Geometry: final body of the model. Coordinates: model frame, mm. Face numbers are marked on the shaded views. A direction names the side the tool comes from. Coordinates: 2 decimals unless noted, no trailing zeros. Order: outer loops, then holes, each group sorted by start corner. A loop starts at its lowest first (then second) coordinate and runs counter-clockwise, first axis right, second up. Notation, with made-up numbers: M 78,22.5 L 131,22.5 A19 cw 131,37.5 Z; hole C 19.5,51 d6. An arc over 180 degrees is marked long. Use CSV: the item, a comma, the result in double quotes. Start each with the question number.
Q1. Mould query, pull axis Y, two halves, no side actions, for the marked faces 4, 5, 6 and 7. Classes: +Y half, -Y half, draft (parallel to the pull), parting line (faces both ways), or undercut.
Q2. Section query B-B, the plane y = -1.5. Output: boundary loops of the cut face in (x, z), and give its area (3 significant figures).
Q3. Section query A-A, the plane x = -17. Output: boundary loops of the cut face in (y, z).
Q4. Access query for the marked faces 1, 2 and 3. Directions: +Z, -Z, +X, -X, +Y, -Y. A direction counts if a zero-diameter tool reaches every point of the face in a straight line with its end or side. Return the directions, or none.
Q5. Ray query, probe 1 along Z at (x, y) = (23, -24); probe 2 along X at (y, z) = (0, 9.25); probe 3 along X at (y, z) = (-14.5, 8.5). Return the intervals inside material, ascending.
Q6. First-contact query: P1, Ø2.5, axis at x = 23, z = 7, coming from the +Y side; P2, Ø1, axis at x = 7.5, z = 1.5, coming from the -Y side; P3, Ø2, axis at x = 12.03, y = 7.16, coming from the -Z side; P4, Ø3, axis at y = 8, z = 8.5, coming from the -X side. Flat tips, straight axial feed; report the tip coordinate or a pass-through.
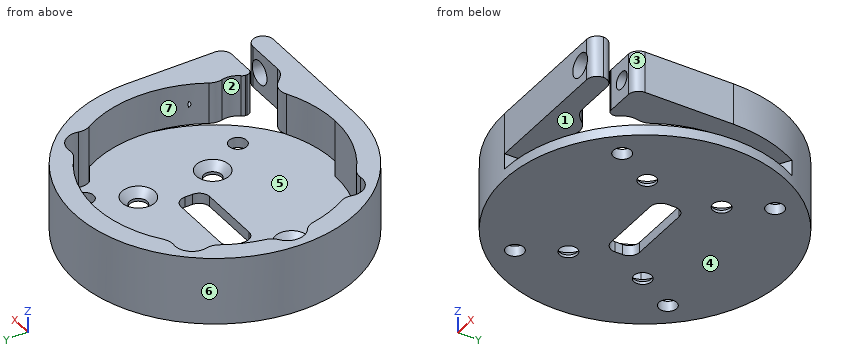
from build123d import *

# Parameters (mm, degrees)
SKETCH_1_R                   = 27
SKETCH_1_R_2                 = 23.1
EXTRUDE_1_DEPTH              = 11
EXTRUDE_START                = 2
SKETCH_2_R                   = 27
EXTRUDE_2_DEPTH              = 2
EXTRUDE_START_2              = -8
EXTRUDE_3_DEPTH              = 8
CUT_EXTRUDE_START            = -8
CUT_EXTRUDE_1_DEPTH          = 8
HOLE_WIZARD_M41_D            = 4.5
HOLE_WIZARD_M41_DEPTH        = 3.9
M4X0_71_D                    = 3.3
M4X0_71_DEPTH                = 10.5
M4X0_71_TIP                  = 0.991420021
CUT_EXTRUDE_START_2          = -3
CUT_EXTRUDE_2_DEPTH          = 3
FILLET_1_R                   = 2
SKETCH_11_W                  = 16
SKETCH_11_H                  = 5.5
CUT_EXTRUDE_3_DEPTH          = 40.736633068
SKETCH_15_R                  = 3.3
SKETCH_15_R_2                = 3.5
CUT_EXTRUDE_5_DEPTH          = 40.736633068
FILLET_3_R                   = 3
SKETCH_16_W                  = 6.088373552
SKETCH_16_H                  = 3.13806494
CUT_EXTRUDE_6_DEPTH          = 11
HOLE_WIZARD_M31_D            = 3.4
HOLE_WIZARD_M31_DEPTH        = 18
HOLE_WIZARD_M31_TIP          = 1.021463052
HOLE_WIZARD_M31_2_AT_2_COUNT = 2
HOLE_WIZARD_M31_2_AT_2_PITCH = 14.310111001
HOLE_WIZARD_M31_2_AT_3_COUNT = 2
HOLE_WIZARD_M31_2_AT_3_PITCH = 28
HOLE_WIZARD_M31_2_AT_4_COUNT = 2
HOLE_WIZARD_M31_2_AT_4_PITCH = 24.067004865
FILLET_7_R                   = 2
EXTRUDE_4_DEPTH              = 8
FILLET_8_R                   = 3
FILLET_9_R                   = 1


with BuildPart() as part:
    # Эскиз1 → Бобышка-Вытянуть1 (new body)
    with BuildSketch(Plane.XY):
        Circle(SKETCH_1_R)
        Circle(SKETCH_1_R_2, mode=Mode.SUBTRACT)
    extrude(amount=EXTRUDE_1_DEPTH)

    # Эскиз2 → Бобышка-Вытянуть2 (add)
    with BuildSketch(Plane(origin=(0, 0, 0), x_dir=(-1, 0, 0), z_dir=(0, 0, -1)).offset(EXTRUDE_START)):
        Circle(SKETCH_2_R)
    extrude(amount=-EXTRUDE_2_DEPTH)

    # Эскиз3 → Бобышка-Вытянуть3 (add)
    with BuildSketch(Plane.XY.offset(11).offset(EXTRUDE_START_2)):
        with BuildLine():
            Line((0, -27), (27, -27))
            Line((27, -27), (27, 0))
            ThreePointArc((27, 0), (19.091883092, -19.091883092), (0, -27))
        make_face()
    extrude(amount=EXTRUDE_3_DEPTH)

    # Эскиз4 → Вырез-Вытянуть1 (cut)
    with BuildSketch(Plane.XY.offset(11).offset(CUT_EXTRUDE_START)):
        with BuildLine():
            Line((0, -23.1), (27, -23.1))
            Line((27, -23.1), (27, -19))
            Line((27, -19), (13.138112498, -19))
            ThreePointArc((13.138112498, -19), (6.88149693, -22.051190444), (0, -23.1))
        make_face()
    extrude(amount=CUT_EXTRUDE_1_DEPTH, mode=Mode.SUBTRACT)

    # Отверстие с зазором M41
    with Locations(Plane(origin=(0, -27, 0), x_dir=(-1, 0, 0), z_dir=(0, -1, 0))):
        with Locations((-23, -7)):
            Hole(HOLE_WIZARD_M41_D / 2, depth=HOLE_WIZARD_M41_DEPTH)

    # Отверстие обработанное метчиком M4x0.71
    with Locations(Plane(origin=(0, -19, 0), x_dir=(-1, 0, 0), z_dir=(0, -1, 0))):
        with Locations((-23, -7)):
            Hole(M4X0_71_D / 2, depth=M4X0_71_DEPTH)
            with Locations((0, 0, -(M4X0_71_DEPTH + M4X0_71_TIP / 2))):  # 118° drill point
                Cone(0, M4X0_71_D / 2, M4X0_71_TIP, mode=Mode.SUBTRACT)

    # Эскиз10 → Вырез-Вытянуть2 (cut)
    with BuildSketch(Plane.XY.offset(3).offset(CUT_EXTRUDE_START_2)):
        with BuildLine():
            Line((20.005186827, 11.55), (23.382685902, 13.5))
            ThreePointArc((23.382685902, 13.5), (23.382685902, -13.5), (0, -27))
            Line((0, -27), (0, -23.1))
            ThreePointArc((0, -23.1), (20.005186827, -11.55), (20.005186827, 11.55))
        make_face()
    extrude(amount=CUT_EXTRUDE_2_DEPTH, mode=Mode.SUBTRACT)

    # Скругление1
    # the kernel refuses this fillet: 2 mm, written as the material it takes off along each edge
    with BuildSketch(Plane(origin=(27, -27, -2), x_dir=(-1, 0, 0), z_dir=(0, 0, 1)), Plane(origin=(27, -19, -2), x_dir=(-1, 0, 0), z_dir=(0, 0, 1))) as fillet_1_piece_1:
        with BuildLine():
            CenterArc((FILLET_1_R, -FILLET_1_R), FILLET_1_R, 90, 90)
            Line((0, -FILLET_1_R), (0, 0))
            Line((0, 0), (FILLET_1_R, 0))
        make_face()
    extrude(amount=18, mode=Mode.SUBTRACT)
    with BuildSketch(Plane(origin=(27, -23.1, -2), x_dir=(-1, 0, 0), z_dir=(0, 0, 1))) as fillet_1_piece_2:
        with BuildLine():
            CenterArc((FILLET_1_R, FILLET_1_R), FILLET_1_R, 180, 90)
            Line((0, FILLET_1_R), (0, 0))
            Line((0, 0), (FILLET_1_R, 0))
        make_face()
    extrude(amount=18, mode=Mode.SUBTRACT)

    # Эскиз11 → Вырез-Вытянуть3 (cut, through all)
    with BuildSketch(Plane.XY):
        Rectangle(SKETCH_11_W, SKETCH_11_H)
    extrude(amount=-CUT_EXTRUDE_3_DEPTH, mode=Mode.SUBTRACT)

    # Эскиз15 → Вырез-Вытянуть5 (cut, through all)
    with BuildSketch(Plane.XY):
        with Locations((-16.349186161, 14.72087334)):
            Circle(SKETCH_15_R)
        with Locations((16.349186161, 14.72087334)):
            Circle(SKETCH_15_R)
        with Locations((16.349186161, -14.72087334)):
            Circle(SKETCH_15_R_2)
        with Locations((-16.349186161, -14.72087334)):
            Circle(SKETCH_15_R)
        with Locations((-22, 0)):
            Circle(SKETCH_15_R)
    extrude(amount=CUT_EXTRUDE_5_DEPTH, mode=Mode.SUBTRACT)

    # Скругление3
    fillet_3_edges = [part.edges().sort_by_distance(p)[0] for p in [
        (-14.874981636, 17.673282698, 5.5),
        (-19.131325578, 12.946133849, 5.5),
        (19.131325578, 12.946133849, 5.5),
        (14.874981636, 17.673282698, 5.5),
        (19.252179639, -12.765718905, 7),
        (-19.131325578, -12.946133849, 5.5),
        (-14.874981636, -17.673282698, 5.5),
        (-22.88, 3.180503105, 5.5),
        (-22.88, -3.180503105, 5.5),
    ]]
    fillet(fillet_3_edges, radius=FILLET_3_R)

    # Эскиз16 → Вырез-Вытянуть6 (cut)
    with BuildSketch(Plane.XY.offset(11)):
        with Locations((15.687994571, -18.137334547)):
            Rectangle(SKETCH_16_W, SKETCH_16_H)
    extrude(amount=-CUT_EXTRUDE_6_DEPTH, mode=Mode.SUBTRACT)

    # Hole Wizard M31
    with Locations(Plane.XY):
        with Locations((-16.349186161, 14.72087334), (16.349186161, 14.72087334), (16.349186161, -14.72087334), (-16.349186161, -14.72087334)):
            Hole(HOLE_WIZARD_M31_D / 2, depth=HOLE_WIZARD_M31_DEPTH)
            with Locations((0, 0, -(HOLE_WIZARD_M31_DEPTH + HOLE_WIZARD_M31_TIP / 2))):  # 118° drill point
                Cone(0, HOLE_WIZARD_M31_D / 2, HOLE_WIZARD_M31_TIP, mode=Mode.SUBTRACT)

    # Эскиз19 → Hole Wizard M31 2 (revolve, cut)
    with BuildSketch(Plane(origin=(-12.033502432, 7.1550555, 0), x_dir=(0, -1, 0), z_dir=(1, 0, 0))):
        Polygon((0, 0), (0, 2), (1.7, 2), (1.7, 1.45), (3.15, 0), align=None)
    hole_wizard_m31_2 = revolve(axis=Axis((-12.033502432, 7.1550555, 6.35), (0, 0, -1)), mode=Mode.SUBTRACT)

    # Hole Wizard M31 2 at 2: Hole Wizard M31 2 ×2
    with Locations(*[(0, -i * HOLE_WIZARD_M31_2_AT_2_PITCH, 0) for i in range(1, HOLE_WIZARD_M31_2_AT_2_COUNT)]):
        add(hole_wizard_m31_2, mode=Mode.SUBTRACT)

    # Hole Wizard M31 2 at 3: Hole Wizard M31 2 ×2
    with Locations(*[Vector(0.859535888020661, -0.5110753928771503, 0) * (i * HOLE_WIZARD_M31_2_AT_3_PITCH) for i in range(1, HOLE_WIZARD_M31_2_AT_3_COUNT)]):
        add(hole_wizard_m31_2, mode=Mode.SUBTRACT)

    # Hole Wizard M31 2 at 4: Hole Wizard M31 2 ×2
    with Locations(*[(i * HOLE_WIZARD_M31_2_AT_4_PITCH, 0, 0) for i in range(1, HOLE_WIZARD_M31_2_AT_4_COUNT)]):
        add(hole_wizard_m31_2, mode=Mode.SUBTRACT)

    # Скругление7
    fillet_7_edges = [part.edges().sort_by_distance(p)[0] for p in [
        (8, 2.75, -1),
        (8, -2.75, -1),
        (-8, -2.75, -1),
        (-8, 2.75, -1),
    ]]
    fillet(fillet_7_edges, radius=FILLET_7_R)

    # Эскиз21 → Бобышка-Вытянуть4 (add)
    with BuildSketch(Plane.XY.offset(11).offset(EXTRUDE_START_2)):
        with BuildLine():
            Line((16.596130054, -23.1), (0, -23.1))
            ThreePointArc((0, -23.1), (6.777628995, -22.083336369), (12.958671938, -19.122835083))
            ThreePointArc((12.958671938, -19.122835083), (14.479457868, -21.383912063), (16.596130054, -23.1))
        make_face()
    extrude(amount=EXTRUDE_4_DEPTH)

    # Скругление8
    fillet_8_edges = [part.edges().sort_by_distance(p)[0] for p in [
        (16.596130054, -23.1, 7),
        (12.958671938, -19.122835083, 7),
    ]]
    fillet(fillet_8_edges, radius=FILLET_8_R)

    # Скругление9
    fillet_9_edges = [part.edges().sort_by_distance(p)[0] for p in [
        (18.732181347, -17.28433466, 7),
        (18.732181347, -19, 7),
    ]]
    fillet(fillet_9_edges, radius=FILLET_9_R)


solid = part.part
Responses:
1,face 4,"draft"
1,face 5,"undercut"
1,face 6,"parting line"
1,face 7,"undercut"
2,outline,"M -26.96,-2 L -7.85,-2 L -7.85,0 L -24.94,0 L -24.94,11 L -26.96,11 Z; M 7.85,-2 L 26.96,-2 L 26.96,0 L 7.85,0 Z; M 23.05,3 L 27,3 L 27,11 L 23.05,11 Z"
2,area,"130 mm²"
3,outline,"M -20.98,-2 L -16.29,-2 L -16.29,0 L -17.96,0 L -17.96,11 L -20.98,11 Z; M -13.15,-2 L 13.15,-2 L 13.15,0 L -13.15,0 Z; M 16.29,-2 L 20.98,-2 L 20.98,11 L 17.96,11 L 17.96,0 L 16.29,0 Z"
4,face 1,"+X, -Y"
4,face 2,"+Z"
4,face 3,"+Z, -Z, +X"
5,probe 1,"z = 3 to 4.75, 9.25 to 11"
5,probe 2,"x = -27 to -25.3, 23.1 to 27"
5,probe 3,"x = -22.78 to -19.64, 19.84 to 22.31, 23.69 to 27"
6,P1,"stops at y = 16"
6,P2,"stops at y = 21.67"
6,P3,"passes through"
6,P4,"stops at x = -26.21"
